Build history of the part. All positions in model axes, mm. Face numbers are marked on the shaded views. A direction names the side the tool comes from. Round coordinates to 2 decimals unless told otherwise and drop trailing zeros. Order: outer loops, then holes, each group sorted by start corner. A loop starts at its lowest first (then second) coordinate and runs counter-clockwise, first axis right, second up. Notation, with made-up numbers: (87.5, 87) -> (145.5, 87) arc R17 ccw to (145.5, 95) -> close; hole circle Ø9 at (59, 6.25). An arc over 180 degrees is marked (long way). Answer as a JSON object with one key per item and string values.
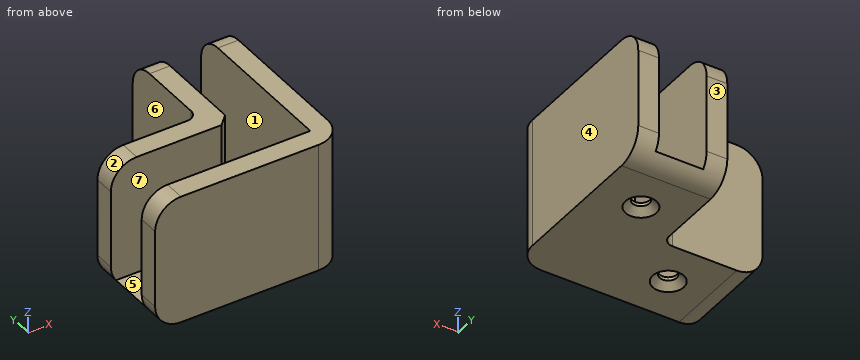
from build123d import *
from build123d import SkipClean  # not in build123d's __all__

# Parameters (mm, degrees)
F1_DEPTH       = 2
F2_DEPTH       = 25
F3_T1_DEPTH    = 29
F3_T3_DEPTH    = 29
F3_T5_DEPTH    = 29
F3_T7_DEPTH    = 29
F3_T9_DEPTH    = 42.2
F3_T11_DEPTH   = 42.2
F3_T13_DEPTH   = 50
F4_R           = 2
F5_SIZE        = 2
F7_D           = 3.3
F7_CSINK_D     = 6
F7_CSINK_ANGLE = 90


# Not quite as in the source:
# - a fillet or chamfer that OpenCascade refuses, or shapes differently, is made with other operations: its cross-section is extruded or revolved along the edge and cut away or added
# - a feature names something its author has since deleted; it is built from what else it names


with BuildPart() as f1:
    # F0 (on Top) → F1 (new body)
    with BuildSketch(Plane.XY):
        Polygon((4.9215265818, 0), (4.9215265818, 9.2), (4.9215265818, 32.5735770881), (-4.2784734182, 32.5735770881), (-4.2784734182, 9.2), (-27.6520505063, 9.2), (-27.6520505063, 0), (0, 0), align=None)
        Polygon((4.9215265818, 32.5735770881), (4.9215265818, 9.2), (4.9215265818, 0), (0, 0), (-27.6520505063, 0), (-27.6520505063, -4), (0, -4), (8.9215265818, -4), (8.9215265818, 32.5735770881), align=None)
        Polygon((-4.2784734182, 9.2), (-4.2784734182, 32.5735770881), (-8.2784734182, 32.5735770881), (-8.2784734182, 13.2), (-27.6520505063, 13.2), (-27.6520505063, 9.2), align=None)
    extrude(amount=F1_DEPTH)

    # F0 (on Top) → F2 (join)
    with BuildSketch(Plane.XY):
        Polygon((-4.2784734182, 9.2), (-4.2784734182, 32.5735770881), (-8.2784734182, 32.5735770881), (-8.2784734182, 13.2), (-27.6520505063, 13.2), (-27.6520505063, 9.2), align=None)
        Polygon((4.9215265818, 32.5735770881), (4.9215265818, 9.2), (4.9215265818, 0), (0, 0), (-27.6520505063, 0), (-27.6520505063, -4), (0, -4), (8.9215265818, -4), (8.9215265818, 32.5735770881), align=None)
    extrude(amount=F2_DEPTH)

    # F3: fillet of radius 5 on 7 edges, made by hand

    # F3_s2 → F3_t1 (cut)
    with BuildSketch(Plane.XZ.offset(-12.5)):
        with BuildLine():
            ThreePointArc((-22.6520505063, 25), (-26.1875844123, 23.5355339059), (-27.6520505063, 20))
            Line((-27.6520505063, 20), (-27.6520505063, 25))
            Line((-27.6520505063, 25), (-22.6520505063, 25))
        make_face()
    extrude(amount=F3_T1_DEPTH, mode=Mode.SUBTRACT)

    # F3_s4 → F3_t3 (cut)
    with BuildSketch(Plane.XZ.offset(-25.7)):
        with BuildLine():
            ThreePointArc((-22.6520505063, 25), (-26.1875844123, 23.5355339059), (-27.6520505063, 20))
            Line((-27.6520505063, 20), (-27.6520505063, 25))
            Line((-27.6520505063, 25), (-22.6520505063, 25))
        make_face()
    extrude(amount=F3_T3_DEPTH, mode=Mode.SUBTRACT)

    # F3_s6 → F3_t5 (cut)
    with BuildSketch(Plane.YZ.offset(-20.7784734182)):
        with BuildLine():
            ThreePointArc((27.5735770881, 25), (31.1091109941, 23.5355339059), (32.5735770881, 20))
            Line((32.5735770881, 20), (32.5735770881, 25))
            Line((32.5735770881, 25), (27.5735770881, 25))
        make_face()
    extrude(amount=F3_T5_DEPTH, mode=Mode.SUBTRACT)

    # F3_s8 → F3_t7 (cut)
    with BuildSketch(Plane.YZ.offset(-7.5784734182)):
        with BuildLine():
            ThreePointArc((32.5735770881, 20), (31.1091109941, 23.5355339059), (27.5735770881, 25))
            Line((27.5735770881, 25), (32.5735770881, 25))
            Line((32.5735770881, 25), (32.5735770881, 20))
        make_face()
    with SkipClean():  # cleaning this boolean's faces spoils the solid; the shape is the same uncleaned
        extrude(amount=F3_T7_DEPTH, mode=Mode.SUBTRACT)

    # F3_s10 → F3_t9 (cut)
    with BuildSketch(Plane.XZ.offset(-25.7)):
        with BuildLine():
            ThreePointArc((-22.6520505063, 0), (-26.1875844123, 1.4644660941), (-27.6520505063, 5))
            Line((-27.6520505063, 5), (-27.6520505063, 0))
            Line((-27.6520505063, 0), (-22.6520505063, 0))
        make_face()
    extrude(amount=F3_T9_DEPTH, mode=Mode.SUBTRACT)

    # F3_s12 → F3_t11 (cut)
    with BuildSketch(Plane.YZ.offset(-20.7784734182)):
        with BuildLine():
            ThreePointArc((27.5735770881, 0), (31.1091109941, 1.4644660941), (32.5735770881, 5))
            Line((32.5735770881, 5), (32.5735770881, 0))
            Line((32.5735770881, 0), (27.5735770881, 0))
        make_face()
    extrude(amount=F3_T11_DEPTH, mode=Mode.SUBTRACT)

    # F3_s14 → F3_t13 (cut)
    with BuildSketch(Plane.XY.offset(-12.5)):
        with BuildLine():
            ThreePointArc((3.9215265818, -4), (7.4570604877, -2.5355339059), (8.9215265818, 1))
            Line((8.9215265818, 1), (8.9215265818, -4))
            Line((8.9215265818, -4), (3.9215265818, -4))
        make_face()
    extrude(amount=F3_T13_DEPTH, mode=Mode.SUBTRACT)

    # F4
    f4_edges = [f1.edges().sort_by_distance(p)[0] for p in [
        (-8.278473, 13.2, 12.5),
    ]]
    fillet(f4_edges, radius=F4_R)

    # F5
    f5_edges = [f1.edges().sort_by_distance(p)[0] for p in [
        (-4.278473, 9.2, 13.5),
    ]]
    chamfer(f5_edges, length=F5_SIZE)

    # F7 (through all)
    with Locations(Plane(origin=(0, 0, 0), x_dir=(1, 0, 0), z_dir=(0, 0, -1))):
        with Locations((-15, -4.6), (0, -19.6)):
            CounterSinkHole(F7_D / 2, F7_CSINK_D / 2, counter_sink_angle=F7_CSINK_ANGLE)


solid = f1.part
1) Cut at C-C, the plane z = 6.25. Give the cut face in (x, y), plus the area to 3 significant figures.
Checked values:
{"outline": "(-27.65, -4) -> (3.92, -4) arc R5 ccw to (8.92, 1) -> (8.92, 32.57) -> (4.92, 32.57) -> (4.92, 0) -> (-27.65, 0) -> close; (-27.65, 9.2) -> (-6.28, 9.2) -> (-4.28, 11.2) -> (-4.28, 32.57) -> (-8.28, 32.57) -> (-8.28, 15.2) arc R2 cw to (-10.28, 13.2) -> (-27.65, 13.2) -> close", "area": "441 mm²"}
2) Cut at A-A, the plane x = 0. Give the cut face in (y, z), plus the area to 3 significant figures.
Checked values:
{"outline": "(-4, 0) -> (16.6, 0) -> (17.95, 1.35) -> (17.95, 2) -> (0, 2) -> (0, 25) -> (-4, 25) -> close; (21.25, 1.35) -> (22.6, 0) -> (27.57, 0) arc R5 ccw to (31.57, 2) -> (21.25, 2) -> close", "area": "152 mm²"}
3) Cut at B-B, the plane y = 4.6. Give the cut face in (x, z), plus the area to 3 significant figures.
Checked values:
{"outline": "(-26.65, 2) arc R5 ccw to (-22.65, 0) -> (-18, 0) -> (-16.65, 1.35) -> (-16.65, 2) -> close; (-13.35, 1.35) -> (-12, 0) -> (8.92, 0) -> (8.92, 25) -> (4.92, 25) -> (4.92, 2) -> (-13.35, 2) -> close", "area": "152 mm²"}
4) Cut at D-D, the plane y = 26. Give the cut face in (x, z).
Checked values:
{"outline": "(-8.28, 0) -> (8.92, 0) -> (8.92, 25) -> (4.92, 25) -> (4.92, 2) -> (-4.28, 2) -> (-4.28, 25) -> (-8.28, 25) -> close"}
5) Which spindle directions (+Z, -Z, +X, -X, +Y, -Y) get a long thin tool onto all of the face, cutting with end or side? Do the marked faces 5, 6 and 7. Say none if no direction does.
Checked values:
{"face 5": "+Z", "face 6": "+Z, -Z, -X, +Y", "face 7": "+Z, -X"}
6) Flat gauge pins, fed straight in: pin 1 Ø14 at (y, z) = (27.5, 7.5) entering from -X; pin 2 Ø14 at (x, z) = (-17.5, 13.5) entering from +Y; pin 3 Ø2 at (x, y) = (-15, 4.6) entering from +Z; pin 4 Ø4.5 at (x, y) = (0, 19.6) entering from +Z. Where does each tip first touch, or does it go through?
Checked values:
{"pin 1": "stops at x = -8.28", "pin 2": "stops at y = 13.2", "pin 3": "passes through", "pin 4": "stops at z = 2"}
7) Pull direction X, two halves, no side cores. Call the marked faces 1, 2, 3 and 4: pulls with the +X half, pulls with the -X half, needs draft (parallel to the pull), parting line crosses it, or undercut.
Checked values:
{"face 1": "undercut", "face 2": "pulls with the -X half", "face 3": "needs draft", "face 4": "pulls with the +X half"}
8) Probe L1, parallel to X at y = 19.6, z = 1.75; L2, parallel to X at y = 29, z = 5.75; L3, parallel to Y at x = -19, z = 20.5. List the from-to ranges inside material, lowest first. Write a range as from..to.
Checked values:
{"L1": "x = -8.28..-1.65, 1.65..8.92", "L2": "x = -8.28..-4.28, 4.92..8.92", "L3": "y = -4..0, 9.2..13.2"}
